from build123d import *

# Parameters (mm, degrees)
BOSS_EXTRUDE1_DEPTH = 12
SKETCH2_R           = 7.5
BOSS_EXTRUDE2_DEPTH = 55


with BuildPart() as part:
    # Sketch1 → Boss-Extrude1 (new body)
    with BuildSketch(Plane(origin=(0, 0, 0), x_dir=(1, 0, 0), z_dir=(0, 1, 0))):
        with BuildLine():
            Line((-85, 160), (85, 160))
            ThreePointArc((85, 160), (102.67766953, 152.67766953), (110, 135))
            Line((110, 135), (110, -135))
            ThreePointArc((110, -135), (102.67766953, -152.67766953), (85, -160))
            Line((85, -160), (-85, -160))
            ThreePointArc((-85, -160), (-102.67766953, -152.67766953), (-110, -135))
            Line((-110, -135), (-110, 135))
            ThreePointArc((-110, 135), (-102.67766953, 152.67766953), (-85, 160))
        make_face()
    extrude(amount=BOSS_EXTRUDE1_DEPTH)

    # Sketch2 → Boss-Extrude2 (add)
    with BuildSketch(Plane(origin=(0, 12, 0), x_dir=(1, 0, 0), z_dir=(0, 1, 0))):
        with BuildLine():
            Line((-22.5, 100), (22.5, 100))
            ThreePointArc((22.5, 100), (29.571067812, 97.071067812), (32.5, 90))
            Line((32.5, 90), (32.5, -90))
            ThreePointArc((32.5, -90), (29.571067812, -97.071067812), (22.5, -100))
            Line((22.5, -100), (-22.5, -100))
            ThreePointArc((-22.5, -100), (-29.571067812, -97.071067812), (-32.5, -90))
            Line((-32.5, -90), (-32.5, 90))
            ThreePointArc((-32.5, 90), (-29.571067812, 97.071067812), (-22.5, 100))
        make_face()
        with Locations(Location((0, 62.5, 0), (0, 0, 270))):
            Circle(SKETCH2_R, mode=Mode.SUBTRACT)
        with Locations(Location((0, -62.5, 0), (0, 0, 270))):
            Circle(SKETCH2_R, mode=Mode.SUBTRACT)
    extrude(amount=BOSS_EXTRUDE2_DEPTH)


solid = part.part
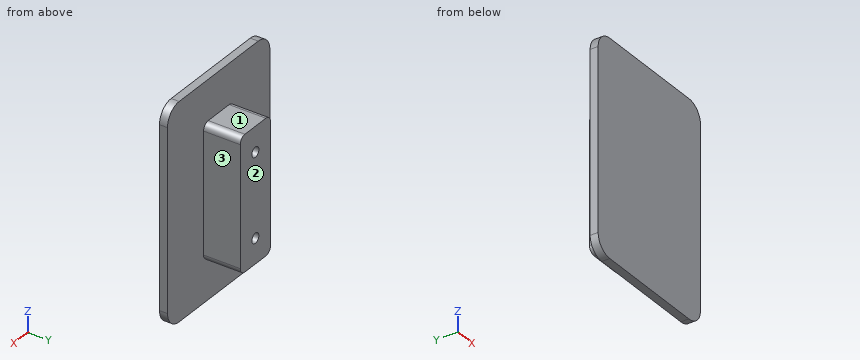
Verification items for the finished model (mm, model axes). Face numbers are marked on the shaded views. A direction names the side the tool comes from. Give positions to 0.01 mm unless a question says otherwise; leave off trailing zeros. Loops run counter-clockwise (first coordinate to the right, second up) from the corner with the lowest first, then second, coordinate; pieces in that order, holes last.
1) Thickness scan on line 1 along X through (y, z) = (38, -62); line 2 along Z through (x, y) = (-4.5, 23); line 3 along X through (y, z) = (41.5, -13). Record the ranges inside material, lowest first.
2) Sectioned sample at C-C, the plane x = 0. Enter the section's corners in (y, z), then the cut area to 3 significant figures.
3) Set-up check for the marked faces 1, 2 and 3: record each of +Z, -Z, +X, -X, +Y, -Y from which the full face is reachable in a straight line by a thin tool's end or side.
4) Sectioned sample at B-B, the plane y = 29.5. Enter the section's corners in (x, z), then the cut area to 3 significant figures.
5) Depth check by flat-ended pin: pin 1 Ø13.5 at (x, y) = (-4.5, 34) entering from -Z; pin 2 Ø4 at (x, z) = (-85, -21.5) entering from -Y; pin 3 Ø13.5 at (x, z) = (0, 62.5) entering from +Y; pin 4 Ø12 at (y, z) = (38, 95) entering from -X. Enter the tip coordinate at first touch or a pass-through.
6) Sectioned sample at D-D, the plane z = 62.5. Enter the section's corners in (x, y), then the cut area to 3 significant figures.
7) Sectioned sample at A-A, the plane z = -50. Enter the section's corners in (x, y).
Answers:
1. line 1: x = -32.5 to -7.48, 7.48 to 32.5
1. line 2: z = -100 to -68.5, -56.5 to 56.5, 68.5 to 100
1. line 3: x = -32.5 to 32.5
2. outline: (0, -160) - (12, -160) - (12, -100) - (67, -100) - (67, -70) - (12, -70) - (12, -55) - (67, -55) - (67, 55) - (12, 55) - (12, 70) - (67, 70) - (67, 100) - (12, 100) - (12, 160) - (0, 160) - close
2. area: 13,200 mm2
3. face 1: +Z, +X, -X, +Y
3. face 2: +Z, -Z, +X, -X, +Y
3. face 3: +Z, -Z, +X, +Y
4. outline: (-32.5, -90) arc R10 ccw to (-22.5, -100) - (22.5, -100) arc R10 ccw to (32.5, -90) - (32.5, 90) arc R10 ccw to (22.5, 100) - (-22.5, 100) arc R10 ccw to (-32.5, 90) - close; hole circle Ø15 at (0, -62.5); hole circle Ø15 at (0, 62.5)
4. area: 12,600 mm2
5. pin 1: stops at z = -100
5. pin 2: stops at y = 0
5. pin 3: stops at y = 12
5. pin 4: stops at x = -32.5
6. outline: (-110, 0) - (110, 0) - (110, 12) - (32.5, 12) - (32.5, 67) - (7.5, 67) - (7.5, 12) - (-7.5, 12) - (-7.5, 67) - (-32.5, 67) - (-32.5, 12) - (-110, 12) - close
6. area: 5,390 mm2
7. outline: (-110, 0) - (110, 0) - (110, 12) - (32.5, 12) - (32.5, 67) - (-32.5, 67) - (-32.5, 12) - (-110, 12) - close
